The drawing under review shows one solid part. Ordinate dimensions are in mm from its lowest x, y, z. Round coordinates to 2 decimals unless told otherwise and drop trailing zeros. Order: outer loops, then holes, each group sorted by start corner. A loop starts at its lowest first (then second) coordinate and runs counter-clockwise, first axis right, second up. Notation, with made-up numbers: M 49,-10 L 76,-10 A23 cw 76,21 Z; hole C 19.25,23.25 d9. An arc over 180 degrees is marked long. Write item = value, one per line. Start each with the question number.
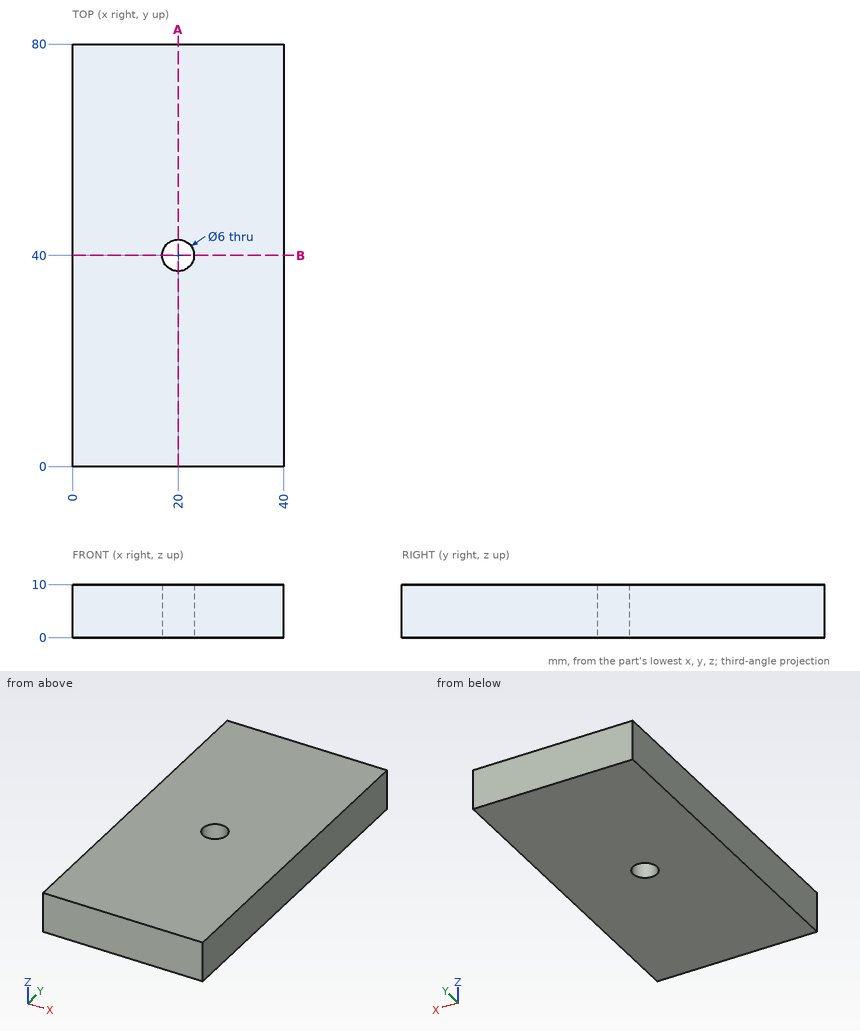
(1) For line 1 along Y through (x, z) = (20, 2); line 2 along X through (y, z) = (40, 8.25); line 3 along X through (y, z) = (39, 8), list the stretches that pass through material, from the lowest coordinate up. Write a range as [from, to].
(2) Insertion check: pin 1 (6 mm diameter, centred on x = 7, z = 7, fed in from -Y); pin 2 (5 mm diameter, centred on x = 20, y = 40, fed in from +Z). Each pin has a flat end and moves straight along its axis. Give the tip position at first contact, or say it passes through.
(3) Consider section B-B, the plane y = 40. Write out the cut boundary in (x, z), then the cut area to 3 significant figures.
(4) Consider section A-A, the plane x = 20. Write out the cut boundary in (y, z), then the cut area to 3 significant figures.
Completed:
q1.line_1 = [0, 37], [43, 80]
q1.line_2 = [0, 17], [23, 40]
q1.line_3 = [0, 17.17], [22.83, 40]
q2.pin_1 = 0
q2.pin_2 = through
q3.outline = M 0,0 L 17,0 L 17,10 L 0,10 Z; M 23,0 L 40,0 L 40,10 L 23,10 Z
q3.area = 340 mm2
q4.outline = M 0,0 L 37,0 L 37,10 L 0,10 Z; M 43,0 L 80,0 L 80,10 L 43,10 Z
q4.area = 740 mm2
